Build history of the part. All positions in model axes, mm. Round coordinates to 2 decimals unless told otherwise and drop trailing zeros. Write each loop counter-clockwise with the first axis right and the second up, starting at its lowest first coordinate (ties: lowest second). Pieces come first, ordered by that corner, then holes. Notation, with made-up numbers: M 36.25,74 L 84.25,74 A10 ccw 84.25,81 Z; hole C 54,5.25 d1. An arc over 180 degrees is marked long. Use a Markdown table: item, result.
from build123d import *

# Parameters (mm, degrees)
SKETCH_1_R      = 1.5
EXTRUDE_1_DEPTH = 3


with BuildPart() as part:
    # 草图1 → 凸台-拉伸1 (new body)
    with BuildSketch(Plane.XY.offset(43)):
        with BuildLine():
            Line((-102, -62), (-8, -62))
            ThreePointArc((-8, -62), (-5.878679656, -61.121320344), (-5, -59))
            Line((-5, -59), (-5, 85))
            ThreePointArc((-5, 85), (-5.878679656, 87.121320344), (-8, 88))
            Line((-8, 88), (-102, 88))
            ThreePointArc((-102, 88), (-104.121320344, 87.121320344), (-105, 85))
            Line((-105, 85), (-105, -59))
            ThreePointArc((-105, -59), (-104.121320344, -61.121320344), (-102, -62))
        make_face()
        with Locations(Location((-94, 71.5, 0), (0, 0, 180))):
            Circle(SKETCH_1_R, mode=Mode.SUBTRACT)
        with Locations(Location((-94, 22.5, 0), (0, 0, 180))):
            Circle(SKETCH_1_R, mode=Mode.SUBTRACT)
        with Locations(Location((-36, 22.5, 0), (0, 0, 180))):
            Circle(SKETCH_1_R, mode=Mode.SUBTRACT)
        with Locations(Location((-36, 71.5, 0), (0, 0, 180))):
            Circle(SKETCH_1_R, mode=Mode.SUBTRACT)
        with Locations(Location((-100.157022476, 13, 0), (0, 0, 180))):
            Circle(SKETCH_1_R, mode=Mode.SUBTRACT)
        with Locations(Location((-12, 81, 0), (0, 0, 180))):
            Circle(SKETCH_1_R, mode=Mode.SUBTRACT)
        with Locations(Location((-98, -55, 0), (0, 0, 180))):
            Circle(SKETCH_1_R, mode=Mode.SUBTRACT)
        with Locations(Location((-98, 81, 0), (0, 0, 180))):
            Circle(SKETCH_1_R, mode=Mode.SUBTRACT)
        with Locations(Location((-12, -55, 0), (0, 0, 180))):
            Circle(SKETCH_1_R, mode=Mode.SUBTRACT)
    extrude(amount=-EXTRUDE_1_DEPTH)


solid = part.part
Q1. Cut at C-C on y = 81. Give the cut face in (x, z), and give its area (3 significant figures).
Response values:
| item | result |
|---|---|
| outline | M -105,40 L -99.5,40 L -99.5,43 L -105,43 Z; M -96.5,40 L -13.5,40 L -13.5,43 L -96.5,43 Z; M -10.5,40 L -5,40 L -5,43 L -10.5,43 Z |
| area | 282 mm2 |
Q2. Cut at A-A on x = -36. Give the cut face in (y, z), and give its area (3 significant figures).
Response values:
| item | result |
|---|---|
| outline | M -62,40 L 21,40 L 21,43 L -62,43 Z; M 24,40 L 70,40 L 70,43 L 24,43 Z; M 73,40 L 88,40 L 88,43 L 73,43 Z |
| area | 432 mm2 |
Q3. Drill centre lines: L1, parallel to X at y = 22.5, z = 41.6; L2, parallel to X at y = 81, z = 40.9; L3, parallel to Y at x = -98, z = 42.3. Where is each one in solid material? Low to high.
Response values:
| item | result |
|---|---|
| L1 | x = -105 to -95.5, -92.5 to -37.5, -34.5 to -5 |
| L2 | x = -105 to -99.5, -96.5 to -13.5, -10.5 to -5 |
| L3 | y = -62 to -56.5, -53.5 to 79.5, 82.5 to 88 |
Q4. Two-plate mould, pull along Y, no slides. Class faces 1 (the cylindrical face through (-34.89, 21.49, 41.52)), 2 (the cylindrical face through (-104.1, 87.14, 41.52)), 3 (the flat face through (-56, 14, 43)), 4 (the cylindrical face through (-10.8, -54.1, 41.5)): +Y half, -Y half, draft (parallel to the pull), parting line (faces both ways), or undercut.
Response values:
| item | result |
|---|---|
| face 1 | undercut |
| face 2 | +Y half |
| face 3 | draft |
| face 4 | undercut |
Q5. Cut at B-B on y = 13. Give the cut face in (x, z).
Response values:
| item | result |
|---|---|
| outline | M -105,40 L -101.66,40 L -101.66,43 L -105,43 Z; M -98.66,40 L -5,40 L -5,43 L -98.66,43 Z |
